Check sheet for the modelled part. Datum: model origin and axes. Units: mm. A direction names the side the tool comes from. Coordinates: 2 decimals unless noted, no trailing zeros. Loops run counter-clockwise (first coordinate to the right, second up) from the corner with the lowest first, then second, coordinate; pieces in that order, holes last. Notation, with made-up numbers: (-17.75, 5) - (-12.75, 5) arc R31 cw to (-12.75, 37) - close; hole circle Ø10 at (-13, 72.5). An arc over 180 degrees is marked (long way). Answer as a JSON object with one key per item and string values. Group by question number.
from build123d import *

# Parameters (mm, degrees)
EXTRUDE_1_DEPTH     = 53
CUT_EXTRUDE_2_REACH = 472.389
SKETCH_2_W          = 75
SKETCH_2_H          = 22
CUT_EXTRUDE_5_REACH = 471.913
SKETCH_4_R          = 2
CUT_EXTRUDE_6_REACH = 471.052
SKETCH_3_W          = 380
SKETCH_3_H          = 22
CUT_EXTRUDE_7_REACH = 470.746
SKETCH_6_W          = 93.868990514
SKETCH_6_H          = 40.944884918
CUT_EXTRUDE_8_DEPTH = 470.912954074


with BuildPart() as part:
    # 草图1 → 凸台-拉伸1 (new body)
    with BuildSketch(Plane(origin=(0, 0, 0), x_dir=(1, 0, 0), z_dir=(0, 1, 0))):
        Polygon((0, 0), (0, 70), (-16, 70), (-16, 465), (-11, 465), (-11, 75), (5, 75), (5, 0), (5, -16.047693785), (-42.239607079, -16.047693785), (-42.239607079, 0), align=None)
    extrude(amount=EXTRUDE_1_DEPTH)

    # 草图2 → 切除-拉伸2 (cut, up to next)
    with BuildSketch(Plane(origin=(5, 0, 0), x_dir=(0, 0, -1), z_dir=(1, 0, 0)), mode=Mode.PRIVATE) as cut_extrude_2_sk1:
        with Locations((37.5, 26.5)):
            Rectangle(SKETCH_2_W, SKETCH_2_H)
    cut_extrude_2_tool1 = extrude(cut_extrude_2_sk1.sketch, amount=-CUT_EXTRUDE_2_REACH, mode=Mode.PRIVATE) & part.part
    add(cut_extrude_2_tool1.solids().sort_by_distance((5, 26.5, -37.5))[0], mode=Mode.SUBTRACT)

    # 草图4 → 切除-拉伸5 (cut, up to next)
    with BuildSketch(Plane.ZY, mode=Mode.PRIVATE) as cut_extrude_5_sk1:
        with Locations((-57, 11.5)):
            Circle(SKETCH_4_R)
    cut_extrude_5_tool1 = extrude(cut_extrude_5_sk1.sketch, amount=-CUT_EXTRUDE_5_REACH, mode=Mode.PRIVATE) & part.part
    # 草图4 → 切除-拉伸5 (cut, up to next)
    with BuildSketch(Plane.ZY, mode=Mode.PRIVATE) as cut_extrude_5_sk2:
        with Locations((-57, 41.5)):
            Circle(SKETCH_4_R)
    cut_extrude_5_tool2 = extrude(cut_extrude_5_sk2.sketch, amount=-CUT_EXTRUDE_5_REACH, mode=Mode.PRIVATE) & part.part
    # 草图4 → 切除-拉伸5 (cut, up to next)
    with BuildSketch(Plane.ZY, mode=Mode.PRIVATE) as cut_extrude_5_sk3:
        with Locations((-29, 11.5)):
            Circle(SKETCH_4_R)
    cut_extrude_5_tool3 = extrude(cut_extrude_5_sk3.sketch, amount=-CUT_EXTRUDE_5_REACH, mode=Mode.PRIVATE) & part.part
    # 草图4 → 切除-拉伸5 (cut, up to next)
    with BuildSketch(Plane.ZY, mode=Mode.PRIVATE) as cut_extrude_5_sk4:
        with Locations((-29, 41.5)):
            Circle(SKETCH_4_R)
    cut_extrude_5_tool4 = extrude(cut_extrude_5_sk4.sketch, amount=-CUT_EXTRUDE_5_REACH, mode=Mode.PRIVATE) & part.part
    add(cut_extrude_5_tool1.solids().sort_by_distance((0, 11.5, -57))[0], mode=Mode.SUBTRACT)
    add(cut_extrude_5_tool2.solids().sort_by_distance((0, 41.5, -57))[0], mode=Mode.SUBTRACT)
    add(cut_extrude_5_tool3.solids().sort_by_distance((0, 11.5, -29))[0], mode=Mode.SUBTRACT)
    add(cut_extrude_5_tool4.solids().sort_by_distance((0, 41.5, -29))[0], mode=Mode.SUBTRACT)

    # 草图3 → 切除-拉伸6 (cut, up to next)
    with BuildSketch(Plane(origin=(-11, 0, 0), x_dir=(0, 0, -1), z_dir=(1, 0, 0)), mode=Mode.PRIVATE) as cut_extrude_6_sk1:
        with Locations((265, 26.5)):
            Rectangle(SKETCH_3_W, SKETCH_3_H)
    cut_extrude_6_tool1 = extrude(cut_extrude_6_sk1.sketch, amount=-CUT_EXTRUDE_6_REACH, mode=Mode.PRIVATE) & part.part
    add(cut_extrude_6_tool1.solids().sort_by_distance((-11, 26.5, -265))[0], mode=Mode.SUBTRACT)

    # 草图5 → 切除-拉伸7 (cut, up to next)
    with BuildSketch(Plane.ZY.offset(16), mode=Mode.PRIVATE) as cut_extrude_7_sk1:
        with BuildLine():
            Line((-143, 8.3), (-113, 8.3))
            ThreePointArc((-113, 8.3), (-110.45, 5.75), (-113, 3.2))
            Line((-113, 3.2), (-143, 3.2))
            ThreePointArc((-143, 3.2), (-145.55, 5.75), (-143, 8.3))
        make_face()
    cut_extrude_7_tool1 = extrude(cut_extrude_7_sk1.sketch, amount=-CUT_EXTRUDE_7_REACH, mode=Mode.PRIVATE) & part.part
    # 草图5 → 切除-拉伸7 (cut, up to next)
    with BuildSketch(Plane.ZY.offset(16), mode=Mode.PRIVATE) as cut_extrude_7_sk2:
        with BuildLine():
            Line((-143, 49.8), (-113, 49.8))
            ThreePointArc((-113, 49.8), (-110.45, 47.25), (-113, 44.7))
            Line((-113, 44.7), (-143, 44.7))
            ThreePointArc((-143, 44.7), (-145.55, 47.25), (-143, 49.8))
        make_face()
    cut_extrude_7_tool2 = extrude(cut_extrude_7_sk2.sketch, amount=-CUT_EXTRUDE_7_REACH, mode=Mode.PRIVATE) & part.part
    # 草图5 → 切除-拉伸7 (cut, up to next)
    with BuildSketch(Plane.ZY.offset(16), mode=Mode.PRIVATE) as cut_extrude_7_sk3:
        with BuildLine():
            Line((-423, 3.25), (-453, 3.25))
            ThreePointArc((-453, 3.25), (-455.5, 5.75), (-453, 8.25))
            Line((-453, 8.25), (-423, 8.25))
            ThreePointArc((-423, 8.25), (-420.5, 5.75), (-423, 3.25))
        make_face()
    cut_extrude_7_tool3 = extrude(cut_extrude_7_sk3.sketch, amount=-CUT_EXTRUDE_7_REACH, mode=Mode.PRIVATE) & part.part
    # 草图5 → 切除-拉伸7 (cut, up to next)
    with BuildSketch(Plane.ZY.offset(16), mode=Mode.PRIVATE) as cut_extrude_7_sk4:
        with BuildLine():
            Line((-423, 44.75), (-453, 44.75))
            ThreePointArc((-453, 44.75), (-455.5, 47.25), (-453, 49.75))
            Line((-453, 49.75), (-423, 49.75))
            ThreePointArc((-423, 49.75), (-420.5, 47.25), (-423, 44.75))
        make_face()
    cut_extrude_7_tool4 = extrude(cut_extrude_7_sk4.sketch, amount=-CUT_EXTRUDE_7_REACH, mode=Mode.PRIVATE) & part.part
    add(cut_extrude_7_tool1.solids().sort_by_distance((-16, 5.75, -128))[0], mode=Mode.SUBTRACT)
    add(cut_extrude_7_tool2.solids().sort_by_distance((-16, 47.25, -128))[0], mode=Mode.SUBTRACT)
    add(cut_extrude_7_tool3.solids().sort_by_distance((-16, 5.75, -438))[0], mode=Mode.SUBTRACT)
    add(cut_extrude_7_tool4.solids().sort_by_distance((-16, 47.25, -438))[0], mode=Mode.SUBTRACT)

    # 草图6 → 切除-拉伸8 (cut, through all)
    with BuildSketch(Plane(origin=(0, 53, 0), x_dir=(1, 0, 0), z_dir=(0, 1, 0))):
        with Locations((-15.853082152, -8.235463886)):
            Rectangle(SKETCH_6_W, SKETCH_6_H)
    extrude(amount=-CUT_EXTRUDE_8_DEPTH, mode=Mode.SUBTRACT)


solid = part.part
1. Sectioned sample at A-A on x = -3.75. Record the cut outline in (y, z).
2. Sectioned sample at C-C on y = 28.5. Record the cut outline in (x, z).
3. Material ranges on line 1 (Y direction, x = -14.5, z = -137.5); line 2 (Y direction, x = 2.8, z = -29); line 3 (Y direction, x = -13.5, z = -414.5), recorded low to high.
4. Release check for a two-part mould opening along Y. For faces 5 (the face through (5, 45, -43)), 6 (the face through (-13, 53, -223)), 7 (the face through (-12, 37.5, -233)) record: released by +Y, released by -Y, zero draft, split by the parting line, or undercut.
5. Sectioned sample at B-B on z = -289. Record the cut outline in (x, y), plus the area to 3 significant figures.
6. Access from +Z, -Z, +X, -X, +Y, -Y to the whole of each face (thin tool, end or side, straight path). Record for faces 1 (the face through (-12, 15.5, -233)), 2 (the face through (-8, 45, -70)), 3 (the face through (-3, 45, -75)), 4 (the face through (5, 8, -43)).
7. Gauge pin test, flat ends, axial feed: pin 1 (4 mm diameter, centred on x = -14, z = -134, fed in from -Y); pin 2 (3 mm diameter, centred on y = 11.5, z = -29, fed in from +X); pin 3 (6 mm diameter, centred on x = -7.5, y = 38, fed in from +Z); pin 4 (4 mm diameter, centred on x = -8, y = 36.5, fed in from -Z). Record the tip position at first contact, or that the pin passes through.
Answers follow:
{
 "1": {"outline": "(0, -75) - (15.5, -75) - (15.5, -70) - (0, -70) - close; (37.5, -75) - (53, -75) - (53, -70) - (37.5, -70) - close"},
 "2": {"outline": "(-16, -465) - (-11, -465) - (-11, -455) - (-16, -455) - close"},
 "3": {"line 1": "y = 0 to 3.2, 8.3 to 15.5, 37.5 to 44.7, 49.8 to 53", "line 2": "y = 0 to 9.5, 13.5 to 15.5, 37.5 to 39.5, 43.5 to 53", "line 3": "y = 0 to 15.5, 37.5 to 53"},
 "4": {"face 5": "zero draft", "face 6": "released by +Y", "face 7": "undercut"},
 "5": {"outline": "(-16, 0) - (-11, 0) - (-11, 15.5) - (-16, 15.5) - close; (-16, 37.5) - (-11, 37.5) - (-11, 53) - (-16, 53) - close", "area": "155 mm^2"},
 "6": {"face 1": "+Z, +X, -X", "face 2": "+Z, -X, +Y, -Y", "face 3": "-Z, +X, +Y, -Y", "face 4": "+Z, -Z, +X, +Y, -Y"},
 "7": {"pin 1": "stops at y = 0", "pin 2": "passes through", "pin 3": "stops at z = -70", "pin 4": "stops at z = -75"}
}
